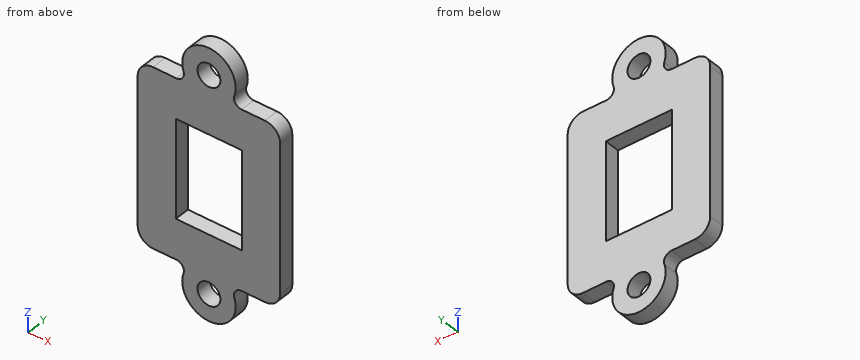
from build123d import *

# Parameters (mm, degrees)
F0_R     = 2.25
F0_W     = 13
F0_H     = 19.3
F1_DEPTH = 3


# Not quite as in the source:
# - a feature names something its author has since deleted; it is built from what else it names


with BuildPart() as f1:
    # F0 (on Front) → F1 (new body)
    with BuildSketch(Plane.XZ):
        with BuildLine():
            Line((-6.4150214341, 17.5), (-11, 17.5))
            ThreePointArc((-11, 17.5), (-13.1213203436, 16.6213203436), (-14, 14.5))
            Line((-14, 14.5), (-14, -14.5))
            ThreePointArc((-14, -14.5), (-13.1213203436, -16.6213203436), (-11, -17.5))
            Line((-11, -17.5), (-6.4150214341, -17.5))
            ThreePointArc((-6.4150214341, -17.5), (-5.200525654, -18.1196591569), (-4.9894611154, -19.4666666667))
            ThreePointArc((-4.9894611154, -19.4666666667), (0, -26.35), (4.9894611154, -19.4666666667))
            ThreePointArc((4.9894611154, -19.4666666667), (5.200525654, -18.1196591569), (6.4150214341, -17.5))
            Line((6.4150214341, -17.5), (11, -17.5))
            ThreePointArc((11, -17.5), (13.1213203436, -16.6213203436), (14, -14.5))
            Line((14, -14.5), (14, 14.5))
            ThreePointArc((14, 14.5), (13.1213203436, 16.6213203436), (11, 17.5))
            Line((11, 17.5), (6.4150214341, 17.5))
            ThreePointArc((6.4150214341, 17.5), (5.200525654, 18.1196591569), (4.9894611154, 19.4666666667))
            ThreePointArc((4.9894611154, 19.4666666667), (0, 26.35), (-4.9894611154, 19.4666666667))
            ThreePointArc((-4.9894611154, 19.4666666667), (-5.200525654, 18.1196591569), (-6.4150214341, 17.5))
        make_face()
        with Locations((0, -21.1)):
            Circle(F0_R, mode=Mode.SUBTRACT)
        Rectangle(F0_W, F0_H, mode=Mode.SUBTRACT)
        with Locations((0, 21.1)):
            Circle(F0_R, mode=Mode.SUBTRACT)
    extrude(amount=F1_DEPTH)


solid = f1.part
Could you check a few things on this model? Use its own coordinates, in mm. Round coordinates to 2 decimals unless told otherwise and drop trailing zeros. Order: outer loops, then holes, each group sorted by start corner. A loop starts at its lowest first (then second) coordinate and runs counter-clockwise, first axis right, second up.
Q1. Please list where these lines run through material, in increasing order: probe 1 along X at (y, z) = (-1.85, -7); probe 2 along Z at (x, y) = (-6.25, -0.5); probe 3 along Z at (x, y) = (10, -2.35).
Geometry says:
probe 1: x = -14 to -6.5, 6.5 to 14
probe 2: z = -17.51 to -9.65, 9.65 to 17.51
probe 3: z = -17.5 to 17.5
Q2. Imagine slicing it at D-D, the plane z = 21.1. List the corners of the cut face in (x, y) for me.
Geometry says:
outline: (-5.25, -3) - (-2.25, -3) - (-2.25, 0) - (-5.25, 0) - close; (2.25, -3) - (5.25, -3) - (5.25, 0) - (2.25, 0) - close
Q3. I'm going to push flat-ended pins straight in: P1, Ø0.9, axis at x = -7.5, y = -2, coming from the +Z side; P2, Ø0.9, axis at x = -9.5, y = -1, coming from the -Z side; P3, Ø1, axis at y = -1.5, z = 15.5, coming from the +X side; P4, Ø2, axis at x = -6.5, z = 19, coming from the -Y side. Where does each tip first touch, or does it pass through?
Geometry says:
P1: stops at z = 17.5
P2: stops at z = -17.5
P3: stops at x = 13.96
P4: passes through
Q4. Imagine slicing it at B-B, the plane x = 0. List the corners of the cut face in (y, z) for me, then the cut area to 3 significant figures.
Geometry says:
outline: (-3, -26.35) - (0, -26.35) - (0, -23.35) - (-3, -23.35) - close; (-3, -18.85) - (0, -18.85) - (0, -9.65) - (-3, -9.65) - close; (-3, 9.65) - (0, 9.65) - (0, 18.85) - (-3, 18.85) - close; (-3, 23.35) - (0, 23.35) - (0, 26.35) - (-3, 26.35) - close
area: 73.2 mm2
Q5. Imagine slicing it at C-C, the plane y = -2.05. List the corners of the cut face in (x, z) for me.
Geometry says:
outline: (-14, -14.5) arc R3 ccw to (-11, -17.5) - (-6.42, -17.5) arc R1.5 cw to (-4.99, -19.47) arc R5.25 ccw (long way) to (4.99, -19.47) arc R1.5 cw to (6.42, -17.5) - (11, -17.5) arc R3 ccw to (14, -14.5) - (14, 14.5) arc R3 ccw to (11, 17.5) - (6.42, 17.5) arc R1.5 cw to (4.99, 19.47) arc R5.25 ccw (long way) to (-4.99, 19.47) arc R1.5 cw to (-6.42, 17.5) - (-11, 17.5) arc R3 ccw to (-14, 14.5) - close; hole (-6.5, -9.65) - (6.5, -9.65) - (6.5, 9.65) - (-6.5, 9.65) - close; hole circle Ø4.5 at (0, -21.1); hole circle Ø4.5 at (0, 21.1)
Q6. Imagine slicing it at A-A, the plane z = -8. List the corners of the cut face in (x, y) for me, then the cut area to 3 significant figures.
Geometry says:
outline: (-14, -3) - (-6.5, -3) - (-6.5, 0) - (-14, 0) - close; (6.5, -3) - (14, -3) - (14, 0) - (6.5, 0) - close
area: 45.0 mm2
